Part model, mm, in its own coordinate system. Round coordinates to 2 decimals unless told otherwise and drop trailing zeros. Loops run counter-clockwise (first coordinate to the right, second up) from the corner with the lowest first, then second, coordinate; pieces in that order, holes last. Notation, with made-up numbers: M -39.75,53.25 L 14.25,53.25 A23 ccw 14.25,73.25 Z; hole C 51,29.5 d2. An arc over 180 degrees is marked long. Write each question's results on one line, items separated by ' | '.
Autodesk Inventor part; units mm, degrees
ref_plane "YZ Plane" through (0, 0, 0) normal (1, 0, 0) x (0, 1, 0)
ref_plane "XZ Plane" through (0, 0, 0) normal (0, 1, 0) x (-1, 0, 0)
ref_plane "XY Plane" through (0, 0, 0) normal (0, 0, 1) x (1, 0, 0)
sketch "Sketch1" plane through (0, 0, 0) normal (0, 0, 1) x (1, 0, 0)
  line L0 (0, 100) -> (0, 50) construction
  line L1 (0, 47) -> (0, 0) construction
  line L2 (0, 50) -> (0, 47) construction
  arc A0 (42, -1970) -> (25, 0) centre (-10972.0978, -1079.9722) ccw
  line L3 (42, -1970) -> (0, -1970)
  line L4 (0, -1970) -> (0, 0)
  line L5 (0, 0) -> (25, 0)
  line L6 (21, 0) -> (39.6023, -210)
  line L7 (39.6023, -210) -> (43.6023, -210)
  dimension "d115" = 3
  dimension "d131" = 11050
  dimension "d132" = 25
  dimension "d133" = 42
  dimension "d134" = 1970
  dimension "d145" = 4
  dimension "d146" = 210
  dimension "d147" = 4
extrude "Plate3" add sketch "Sketch1" along normal blind 3 contours L3 L4 L5 L6 L7 A0
sketch "Sketch3" plane through (0, 0, 0) normal (0, 0, -1) x (-1, 0, 0)
  line L0 (0, 0) -> (0, -1970)
  line L1 (-21, 0) -> (0, 0)
  arc A0 (-43.6023, -210) -> (-42, -1970) centre (10972.0978, -1079.9722) ccw
  line L2 (0, -1970) -> (-42, -1970)
  circle A1 centre (-8, -1950) radius 3.5
  circle A2 centre (0, -1947.1277) radius 5
  circle A3 centre (0, -1947.1277) radius 12
  line L3 (-39.6023, -210) -> (-21, 0)
  line L4 (-43.6023, -210) -> (-39.6023, -210)
  point P0 (0, -1935.1277)
  point P1 (-11.2941, -1951.1827)
  point P2 (-4.7059, -1948.8173)
  point P3 (0, -1942.1277)
  dimension "d135" = 7
  dimension "d136" = 8
  dimension "d137" = 20
  dimension "d143" = 10
extrude "Extrusion2" cut sketch "Sketch3" against normal blind 10 contours A1
pattern_linear "Rectangular Pattern1" count 31 spacing 70 along (0, 1, 0) of "Extrusion2"
equation "\"BendReliefWidth\" = Thickness"
equation "\"BendReliefDepth\" = 0.5 * Thickness"
equation "\"CornerReliefSize\" = 4 * Thickness"
equation "\"MinimumRemnant\" = 2 * Thickness"
equation "\"GapSize\" = Thickness"
properties part number "MSC 084 wall support gills" material "AISI304"
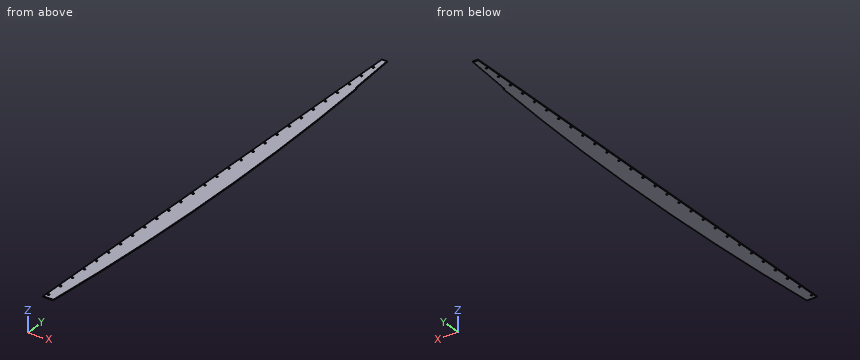
Item 1: Wall check: L1, parallel to X at y = -1092, z = 0.2; L2, parallel to X at y = -1950, z = 1.55; L3, parallel to X at y = -1110, z = 2.3. Give the ranges that are in metal, low to high.
Filled sheet:
L1: 0 to 77.9 | L2: 0 to 4.5, 11.5 to 43.6 | L3: 0 to 4.5, 11.5 to 77.86
Item 2: Band-saw the part on B-B on y = -525.5. Give the cut face in (x, z).
Filled sheet:
outline: M 0,0 L 63.98,0 L 63.98,3 L 0,3 Z
Item 3: Band-saw the part on A-A on z = 2.2. Count the separate pieces of the cut face and the enclosed holes in it, and give its area (3 significant figures).
Filled sheet:
separate pieces: 1 | enclosed holes: 28 | area: 122,000 mm^2
